CAD build for the part. Positions are in the model's coordinates, mm. Face numbers are marked on the shaded views. A direction names the side the tool comes from. Round coordinates to 2 decimals unless told otherwise and drop trailing zeros. Write each loop counter-clockwise with the first axis right and the second up, starting at its lowest first coordinate (ties: lowest second). Pieces come first, ordered by that corner, then holes. Notation, with made-up numbers: (64.5, 16.25) -> (118.5, 16.25) arc R20 ccw to (118.5, 27.25) -> close; hole circle Ø8 at (73, 59.25). An arc over 180 degrees is marked (long way). Put each result on its own line as item: value. Start each with the question number.
1. 3-axis set-ups, long thin cutter, end or side, ignore diameter. For the marked faces 1 and 2: which of +Z, -Z, +X, -X, +Y, -Y reach the whole face in a straight line?
2. Drill centre lines: line 1 (Y direction, x = -6.5, z = 57); line 2 (Z direction, x = 17.5, y = -49). Where is each one in solid material? Low to high. Write a range as from..to.
3. Flat gauge pins, fed straight in: P1, Ø1.5, axis at x = 19.5, y = -9.5, coming from the -Z side; P2, Ø8, axis at x = -19, y = 7.5, coming from the +Z side. Where does each tip first touch, or does it go through?
4. Saw through at A-A on z = 109. List the corners of the cut face in (x, y), and give its area (4 significant figures).
5. Pull direction X, two halves, no side cores. Call the marked faces 3, 4 and 5: pulls with the +X half, pulls with the -X half, needs draft (parallel to the pull), parting line crosses it, or undercut.
6. Saw through at B-B on x = 23. List the corners of the cut face in (y, z).
from build123d import *

# Parameters (mm, degrees)
F0_W     = 120
F0_H     = 120
F1_DEPTH = 120
F2_T     = -2.5
F3_SIZE  = 2


with BuildPart() as f1:
    # F0 (on Top) → F1 (new body)
    with BuildSketch(Plane.XY):
        Rectangle(F0_W, F0_H)
    extrude(amount=F1_DEPTH)

    # F2
    f2_openings = [f1.faces().sort_by_distance(p)[0] for p in [
        (0, 0, 120),
    ]]
    offset(amount=F2_T, openings=f2_openings)

    # F3
    f3_edges = [f1.edges().sort_by_distance(p)[0] for p in [
        (0, 57.5, 120),
        (-57.5, 0, 120),
        (0, -57.5, 120),
        (57.5, 0, 120),
    ]]
    chamfer(f3_edges, length=F3_SIZE)


solid = f1.part
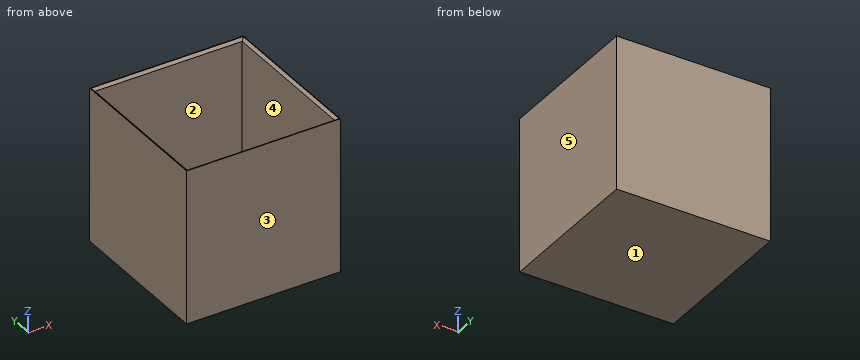
Return value:
1. face 1: -Z, +X, -X, +Y, -Y
1. face 2: +Z
2. line 1: y = -60..-57.5, 57.5..60
2. line 2: z = 0..2.5
3. P1: stops at z = 0
3. P2: stops at z = 2.5
4. outline: (-60, -60) -> (60, -60) -> (60, 60) -> (-60, 60) -> close; hole (-57.5, -57.5) -> (57.5, -57.5) -> (57.5, 57.5) -> (-57.5, 57.5) -> close
4. area: 1,175 mm^2
5. face 3: needs draft
5. face 4: undercut
5. face 5: pulls with the +X half
6. outline: (-60, 0) -> (60, 0) -> (60, 120) -> (59.5, 120) -> (57.5, 118) -> (57.5, 2.5) -> (-57.5, 2.5) -> (-57.5, 118) -> (-59.5, 120) -> (-60, 120) -> close
